The drawing under review shows one solid part. Ordinate dimensions are in mm from its lowest x, y, z. A direction names the side the tool comes from. Coordinates: 2 decimals unless noted, no trailing zeros. Order: outer loops, then holes, each group sorted by start corner. A loop starts at its lowest first (then second) coordinate and runs counter-clockwise, first axis right, second up.
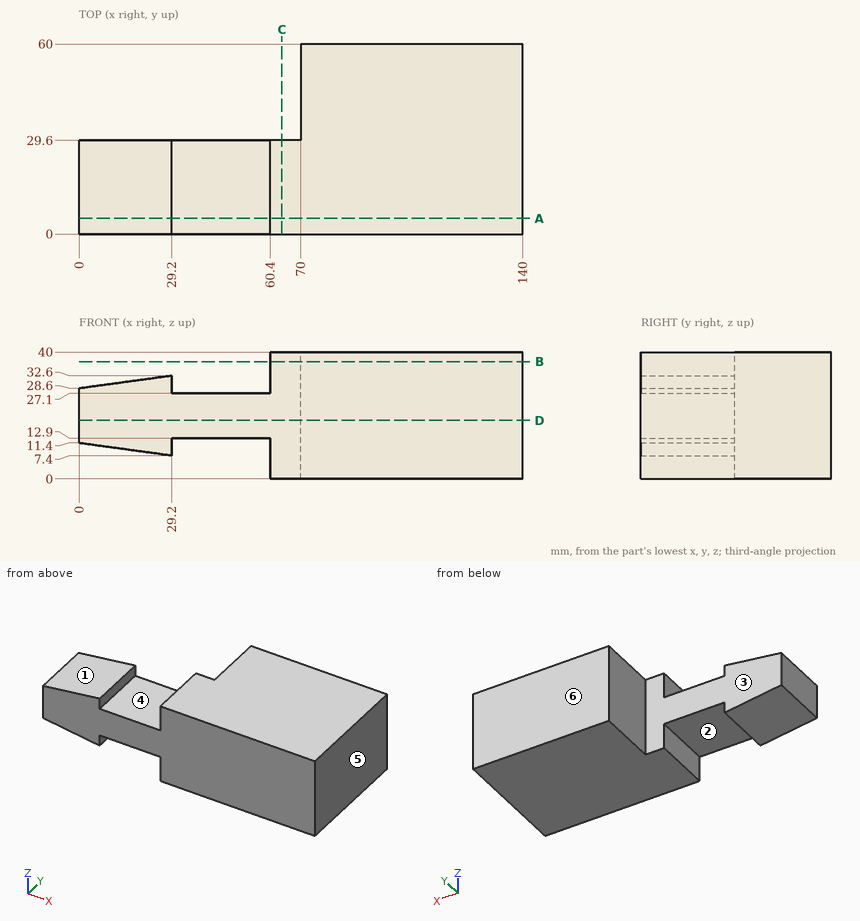
(1) We need section D-D, the plane z = 18.5. Write out the cut boundary in (x, y).
A:
outline: (0, 0) - (140, 0) - (140, 60) - (70, 60) - (70, 29.6) - (0, 29.6) - close
(2) We need section C-C, the plane x = 64. Write out the cut boundary in (y, z), and give its area (3 significant figures).
A:
outline: (0, 0) - (29.6, 0) - (29.6, 40) - (0, 40) - close
area: 1,180 mm2
(3) Draft analysis for pull direction X (two halves, no side actions). For the marked faces 4, 5 and 6, state which applies: released by +X, released by -X, zero draft, split by the parting line, or undercut.
A:
face 4: undercut
face 5: released by +X
face 6: zero draft
(4) We need section B-B, the plane z = 37. Write out the cut boundary in (x, y), and give its area (3 significant figures).
A:
outline: (60.4, 0) - (140, 0) - (140, 60) - (70, 60) - (70, 29.6) - (60.4, 29.6) - close
area: 4,480 mm2
(5) We need section A-A, the plane y = 5. Write out the cut boundary in (x, z).
A:
outline: (0, 11.4) - (29.2, 7.4) - (29.2, 12.9) - (60.4, 12.9) - (60.4, 0) - (140, 0) - (140, 40) - (60.4, 40) - (60.4, 27.1) - (29.2, 27.1) - (29.2, 32.6) - (0, 28.6) - close
(6) Machinability: for the marked faces 1, 2 and 3, which of the approach directions +Z, -Z, +X, -X, +Y, -Y give a long, thin tool a straight path to every point of the face, cutting with its end or side? Answer none if there is none.
A:
face 1: +Z, -X, +Y, -Y
face 2: -Z, +Y, -Y
face 3: +Z, -Z, -X, +Y
(7) Wall thickness on probe 1 along X at (y, z) = (47, 30); probe 2 along Z at (x, y) = (41, 5); probe 3 along X at (y, z) = (3.5, 35.5): over which ranges is each line inside the solid? List them lowest first.
A:
probe 1: x = 70 to 140
probe 2: z = 12.9 to 27.1
probe 3: x = 60.4 to 140
(8) For pin 1 Ø9 at (x, y) = (43, 14.5) entering from -Z; pin 2 Ø10 at (x, z) = (37, 9.5) entering from -Y; pin 3 Ø9 at (x, y) = (48.5, 21.5) entering from +Z; pin 4 Ø2 at (y, z) = (37, 22.5) entering from -X, all flat-tipped, find the tip position at first contact; note any pin that passes through.
A:
pin 1: stops at z = 12.9
pin 2: stops at y = 0
pin 3: stops at z = 27.1
pin 4: stops at x = 70
